```python
from build123d import *

# Parameters (mm, degrees)
F0_W     = 54.485863
F0_H     = 19.160416
F0_R     = 6.40756
F1_DEPTH = 125.30254
F2_R     = 8.789693


with BuildPart() as f1:
    # F0 (on Front) → F1 (new body)
    with BuildSketch(Plane.XZ):
        with Locations((1.870436, -44.420557)):
            Rectangle(F0_W, F0_H)
        with Locations((0, -43.069407)):
            Circle(F0_R, mode=Mode.SUBTRACT)
    extrude(amount=F1_DEPTH)

    # F2
    f2_edges = [f1.edges().sort_by_distance(p)[0] for p in [
        (-25.372496, -62.65127, -34.840349),
    ]]
    fillet(f2_edges, radius=F2_R)


solid = f1.part
```
The model under review builds one solid part; all positions refer to its coordinate system, in mm. Give positions to 0.01 mm unless a question says otherwise; leave off trailing zeros. Write each loop counter-clockwise with the first axis right and the second up, starting at its lowest first coordinate (ties: lowest second). Pieces come first, ordered by that corner, then holes.
(1) Consider section A-A, the plane x = 0. Give the boundary of the cut face in (y, z), and give its area (3 significant figures).
(2) Consider section B-B, the plane y = -109.5. Give the boundary of the cut face in (x, z), and give its area (3 significant figures).
(3) For P1, Ø6, axis at x = 6, z = -46.5, coming from the +Y side, flat-tipped, find the tip position at first contact; note if it passes through.
(4) The part is to be moulded in two halves that separate along Z. For faces 1 (the cylindrical face through (-1.389, -61.774, -49.325)), 2 (the flat face through (8, 0, -44)), 3 (the flat face through (6, -62, -34.84)), say which applies: released by +Z, released by -Z, zero draft, split by the parting line, or undercut.
(5) To check wall thickness, follow L1, parallel to Z at x = 0, y = -85; L2, parallel to X at y = -38, z = -47; L3, parallel to X at y = -98.5, z = -38. State the ranges of each line that lie inside material, in increasing order.
Returned:
1. outline: (-125.3, -54) - (0, -54) - (0, -49.48) - (-125.3, -49.48) - close; (-125.3, -36.66) - (0, -36.66) - (0, -34.84) - (-125.3, -34.84) - close
1. area: 795 mm2
2. outline: (-25.37, -54) - (29.11, -54) - (29.11, -34.84) - (-16.58, -34.84) arc R8.79 ccw to (-25.37, -43.63) - close; hole circle Ø12.82 at (0, -43.07)
2. area: 898 mm2
3. P1: stops at y = 0
4. face 1: undercut
4. face 2: zero draft
4. face 3: released by +Z
5. L1: z = -54 to -49.48, -36.66 to -34.84
5. L2: x = -25.37 to -5.06, 5.06 to 29.11
5. L3: x = -23.33 to -3.92, 3.92 to 29.11
